```python
from build123d import *

# Parameters (mm, degrees)
BASE_FLANGE1_DEPTH  = 1613
FILLET1_R           = 3
CUT_EXTRUDE1_REACH  = 1625.966
SKETCH6_R           = 11
LPATTERN1_COUNT     = 3
LPATTERN1_PITCH     = 132
CUT_EXTRUDE4_REACH  = 1634.045
SKETCH10_R          = 3.25
LPATTERN5_COUNT     = 4
LPATTERN5_PITCH     = 529
CUT_EXTRUDE5_REACH  = 1623.619
CUT_EXTRUDE6_REACH  = 1623.619
SKETCH13_R          = 3.25
CUT_EXTRUDE7_REACH  = 1623.619
SKETCH14_R          = 3.25
LPATTERN6_COUNT     = 3
LPATTERN6_PITCH     = 529
CUT_EXTRUDE8_REACH  = 1623.619
SKETCH15_R          = 3.25
CUT_EXTRUDE9_REACH  = 1623.619
SKETCH16_R          = 3.25
CUT_EXTRUDE10_REACH = 1625.966


# Sheet-metal steps are written as plain solids
with BuildPart() as part:
    # Sketch1 → Base-Flange1 (new body)
    with BuildSketch(Plane(origin=(0, 0, 0), x_dir=(1, 0, 0), z_dir=(0, 1, 0))):
        with BuildLine():
            Line((-113, 149), (-113, 123))
            ThreePointArc((-113, 123), (-112.707106781, 122.292893219), (-112, 122))
            Line((-112, 122), (-61.506905499, 122))
            ThreePointArc((-61.506905499, 122), (-60.303378662, 121.597348789), (-59.584453364, 120.551523153))
            Line((-59.584453364, 120.551523153), (-25.207773318, 0.724238423))
            ThreePointArc((-25.207773318, 0.724238423), (-24.848310669, 0.201325606), (-24.246547251, 0))
            Line((-24.246547251, 0), (24.246547251, 0))
            ThreePointArc((24.246547251, 0), (24.848310669, 0.201325606), (25.207773318, 0.724238423))
            Line((25.207773318, 0.724238423), (59.584453364, 120.551523153))
            ThreePointArc((59.584453364, 120.551523153), (60.303378662, 121.597348789), (61.506905499, 122))
            Line((61.506905499, 122), (87, 122))
            ThreePointArc((87, 122), (87.707106781, 122.292893219), (88, 123))
            Line((88, 123), (88, 149))
            Line((88, 149), (89, 149))
            Line((89, 149), (89, 123))
            ThreePointArc((89, 123), (88.414213562, 121.585786438), (87, 121))
            Line((87, 121), (61.506905499, 121))
            ThreePointArc((61.506905499, 121), (60.90514208, 120.798674394), (60.545679431, 120.275761577))
            Line((60.545679431, 120.275761577), (26.168999386, 0.448476847))
            ThreePointArc((26.168999386, 0.448476847), (25.450074087, -0.597348789), (24.246547251, -1))
            Line((24.246547251, -1), (-24.246547251, -1))
            ThreePointArc((-24.246547251, -1), (-25.450074087, -0.597348789), (-26.168999386, 0.448476847))
            Line((-26.168999386, 0.448476847), (-60.545679431, 120.275761577))
            ThreePointArc((-60.545679431, 120.275761577), (-60.90514208, 120.798674394), (-61.506905499, 121))
            Line((-61.506905499, 121), (-112, 121))
            ThreePointArc((-112, 121), (-113.414213562, 121.585786438), (-114, 123))
            Line((-114, 123), (-114, 149))
            Line((-114, 149), (-113, 149))
        make_face()
    extrude(amount=BASE_FLANGE1_DEPTH)

    # Fillet1
    fillet1_edges = [part.edges().sort_by_distance(p)[0] for p in [
        (-113.5, 0, -149),
        (88.5, 0, -149),
        (-113.5, 1613, -149),
        (88.5, 1613, -149),
    ]]
    fillet(fillet1_edges, radius=FILLET1_R)

    # Sketch6 → Cut-Extrude1 (cut, up to next)
    with BuildSketch(Plane.XY.offset(1), mode=Mode.PRIVATE) as cut_extrude1_sk1:
        with Locations((0, 50)):
            Circle(SKETCH6_R)
    cut_extrude1_tool1 = extrude(cut_extrude1_sk1.sketch, amount=-CUT_EXTRUDE1_REACH, mode=Mode.PRIVATE) & part.part
    cut_extrude1 = cut_extrude1_tool1.solids().sort_by_distance((0, 50, 1))[0]
    add(cut_extrude1, mode=Mode.SUBTRACT)

    # LPattern1: Cut-Extrude1 ×3
    with Locations(*[(0, i * LPATTERN1_PITCH, 0) for i in range(1, LPATTERN1_COUNT)]):
        add(cut_extrude1, mode=Mode.SUBTRACT)

    # Cut-Extrude4: up to this face of the body (flat: up to its plane)
    cut_extrude4_end = Plane(part.part.faces().sort_by_distance((-114, 806.5, -135.998864211))[0])
    # Sketch10 → Cut-Extrude4 (cut, up to the picked face)
    with BuildSketch(Plane(origin=(89, 0, -5.5), x_dir=(0, 0, -1), z_dir=(1, 0, 0)), mode=Mode.PRIVATE) as cut_extrude4_sk1:
        with Locations((133.5, 13)):
            Circle(SKETCH10_R)
    cut_extrude4_tool1 = split(extrude(cut_extrude4_sk1.sketch, amount=-CUT_EXTRUDE4_REACH, mode=Mode.PRIVATE), bisect_by=cut_extrude4_end, keep=Keep.BOTH, mode=Mode.PRIVATE)
    cut_extrude4 = cut_extrude4_tool1.solids().sort_by(Axis((89, 13, -139), (-1, 0, 0)))[0]
    add(cut_extrude4, mode=Mode.SUBTRACT)

    # LPattern5: Cut-Extrude4 ×4
    with Locations(*[(0, i * LPATTERN5_PITCH, 0) for i in range(1, LPATTERN5_COUNT)]):
        add(cut_extrude4, mode=Mode.SUBTRACT)

    # Sketch12 → Cut-Extrude5 (cut, up to next)
    with BuildSketch(Plane.XY.offset(-121), mode=Mode.PRIVATE) as cut_extrude5_sk1:
        with BuildLine():
            Line((-70.006905499, 1447), (-70.006905499, 1417))
            ThreePointArc((-70.006905499, 1417), (-85.006905499, 1402), (-100.006905499, 1417))
            Line((-100.006905499, 1417), (-100.006905499, 1447))
            ThreePointArc((-100.006905499, 1447), (-85.006905499, 1462), (-70.006905499, 1447))
        make_face()
    cut_extrude5_tool1 = extrude(cut_extrude5_sk1.sketch, amount=-CUT_EXTRUDE5_REACH, mode=Mode.PRIVATE) & part.part
    add(cut_extrude5_tool1.solids().sort_by_distance((-85.006905, 1432, -121))[0], mode=Mode.SUBTRACT)

    # Sketch13 → Cut-Extrude6 (cut, up to next)
    with BuildSketch(Plane.XY.offset(-121), mode=Mode.PRIVATE) as cut_extrude6_sk1:
        with Locations((-86.506905499, 25)):
            Circle(SKETCH13_R)
    cut_extrude6_tool1 = extrude(cut_extrude6_sk1.sketch, amount=-CUT_EXTRUDE6_REACH, mode=Mode.PRIVATE) & part.part
    cut_extrude6 = cut_extrude6_tool1.solids().sort_by_distance((-86.506905, 25, -121))[0]
    add(cut_extrude6, mode=Mode.SUBTRACT)

    # Sketch14 → Cut-Extrude7 (cut, up to next)
    with BuildSketch(Plane.XY.offset(-121), mode=Mode.PRIVATE) as cut_extrude7_sk1:
        with Locations((74.006905499, 25)):
            Circle(SKETCH14_R)
    cut_extrude7_tool1 = extrude(cut_extrude7_sk1.sketch, amount=-CUT_EXTRUDE7_REACH, mode=Mode.PRIVATE) & part.part
    cut_extrude7 = cut_extrude7_tool1.solids().sort_by_distance((74.006905, 25, -121))[0]
    add(cut_extrude7, mode=Mode.SUBTRACT)

    # LPattern6: Cut-Extrude6, Cut-Extrude7 ×3
    with Locations(*[(0, i * LPATTERN6_PITCH, 0) for i in range(1, LPATTERN6_COUNT)]):
        add(cut_extrude6, mode=Mode.SUBTRACT)
        add(cut_extrude7, mode=Mode.SUBTRACT)

    # Sketch15 → Cut-Extrude8 (cut, up to next)
    with BuildSketch(Plane.XY.offset(-121), mode=Mode.PRIVATE) as cut_extrude8_sk1:
        with Locations((-86.506905499, 1588)):
            Circle(SKETCH15_R)
    cut_extrude8_tool1 = extrude(cut_extrude8_sk1.sketch, amount=-CUT_EXTRUDE8_REACH, mode=Mode.PRIVATE) & part.part
    add(cut_extrude8_tool1.solids().sort_by_distance((-86.506905, 1588, -121))[0], mode=Mode.SUBTRACT)

    # Sketch16 → Cut-Extrude9 (cut, up to next)
    with BuildSketch(Plane.XY.offset(-121), mode=Mode.PRIVATE) as cut_extrude9_sk1:
        with Locations((74.006905499, 1588)):
            Circle(SKETCH16_R)
    cut_extrude9_tool1 = extrude(cut_extrude9_sk1.sketch, amount=-CUT_EXTRUDE9_REACH, mode=Mode.PRIVATE) & part.part
    add(cut_extrude9_tool1.solids().sort_by_distance((74.006905, 1588, -121))[0], mode=Mode.SUBTRACT)

    # Sketch17 → Cut-Extrude10 (cut, up to next)
    with BuildSketch(Plane.XY.offset(1), mode=Mode.PRIVATE) as cut_extrude10_sk1:
        with BuildLine():
            Line((15, 1518), (15, 1358))
            ThreePointArc((15, 1358), (0, 1343), (-15, 1358))
            Line((-15, 1358), (-15, 1518))
            ThreePointArc((-15, 1518), (0, 1533), (15, 1518))
        make_face()
    cut_extrude10_tool1 = extrude(cut_extrude10_sk1.sketch, amount=-CUT_EXTRUDE10_REACH, mode=Mode.PRIVATE) & part.part
    add(cut_extrude10_tool1.solids().sort_by_distance((0, 1438, 1))[0], mode=Mode.SUBTRACT)


solid = part.part
```
Design review of the part built by this model. Coordinates are the model's own, in mm. A direction names the side the tool comes from. Round coordinates to 2 decimals unless told otherwise and drop trailing zeros. Order: outer loops, then holes, each group sorted by start corner. A loop starts at its lowest first (then second) coordinate and runs counter-clockwise, first axis right, second up. Notation, with made-up numbers: M 81.25,-27 L 89.25,-27 A19 cw 89.25,-5 Z; hole C 8.25,19.5 d1. An arc over 180 degrees is marked long. Put each result on its own line as item: value.
Q1. Machinability: for faces 1 (the face through (74, 795, -122)), 2 (the face through (-86, 795, -121)), 3 (the face through (74, 795, -121)), which of the approach directions +Z, -Z, +X, -X, +Y, -Y give a long, thin tool a straight path to every point of the face, cutting with its end or side? Answer none if there is none.
Reported:
face 1: -Z, +Y, -Y
face 2: +Z, -X, +Y, -Y
face 3: +Z, +X, +Y, -Y
Q2. Consider section C-C (x = -41). State the section outline as (y, z) points.
Reported:
outline: M 0,-55.77 L 1613,-55.77 L 1613,-52.15 L 0,-52.15 Z
Q3. Consider section B-B (y = 1130). State the section outline as (x, z) points.
Reported:
outline: M -114,-149 L -113,-149 L -113,-123 A1 cw -112,-122 L -61.51,-122 A2 ccw -59.58,-120.55 L -25.21,-0.72 A1 cw -24.25,0 L 24.25,0 A1 cw 25.21,-0.72 L 59.58,-120.55 A2 ccw 61.51,-122 L 87,-122 A1 cw 88,-123 L 88,-149 L 89,-149 L 89,-123 A2 ccw 87,-121 L 61.51,-121 A1 cw 60.55,-120.28 L 26.17,-0.45 A2 ccw 24.25,1 L -24.25,1 A2 ccw -26.17,-0.45 L -60.55,-120.28 A1 cw -61.51,-121 L -112,-121 A2 ccw -114,-123 Z
Q4. Draft analysis for pull direction X (two halves, no side actions). For faces 4 (the face through (0, 795, 0)), 5 (the face through (89, 795, -136)), 6 (the face through (-114, 795, -136)), state which applies: released by +X, released by -X, zero draft, split by the parting line, or undercut.
Reported:
face 4: undercut
face 5: released by +X
face 6: released by -X
Q5. Insertion check: pin 1 Ø20.5 at (x, y) = (77, 672.5) entering from +Z; pin 2 Ø10.5 at (y, z) = (542, -139) entering from -X; pin 3 Ø8.5 at (x, y) = (-86.51, 1588) entering from -Z; pin 4 Ø1.5 at (y, z) = (1162.5, -20.5) entering from -X. Each pin has a flat end and moves straight along its axis. Give the tip position at first contact, or say it passes through.
Reported:
pin 1: z = -121
pin 2: x = -114
pin 3: z = -122
pin 4: x = -32.14
Q6. To check wall thickness, follow line 1 (Z direction, x = 88.5, y = 1071); line 2 (Z direction, x = 22, y = 670.5); line 3 (X direction, y = 865.5, z = -60.5). State the ranges of each line that lie inside material, in increasing order.
Reported:
line 1: -149 to -142.25, -135.75 to -121.68
line 2: 0 to 1
line 3: -43.4 to -42.36, 42.36 to 43.4
Q7. Consider section A-A (z = -33). State the section outline as (x, y) points, and give its area (3 significant figures).
Reported:
outline: M -35.51,0 L -34.47,0 L -34.47,1613 L -35.51,1613 Z; M 34.47,0 L 35.51,0 L 35.51,1613 L 34.47,1613 Z
area: 3,360 mm²
